Here's the drawing with two shaded views (mm, measured from the low corner). I have some questions. A direction names the side the tool comes from. Round coordinates to 2 decimals unless told otherwise and drop trailing zeros. Loops run counter-clockwise (first coordinate to the right, second up) from the corner with the lowest first, then second, coordinate; pieces in that order, holes last. Notation, with made-up numbers: (52.25, -38.5) - (109.25, -38.5) arc R11 cw to (109.25, -34.5) - close; hole circle Ø10 at (-25, 75). An arc over 180 degrees is marked (long way). Answer as CSV lines item,"result".
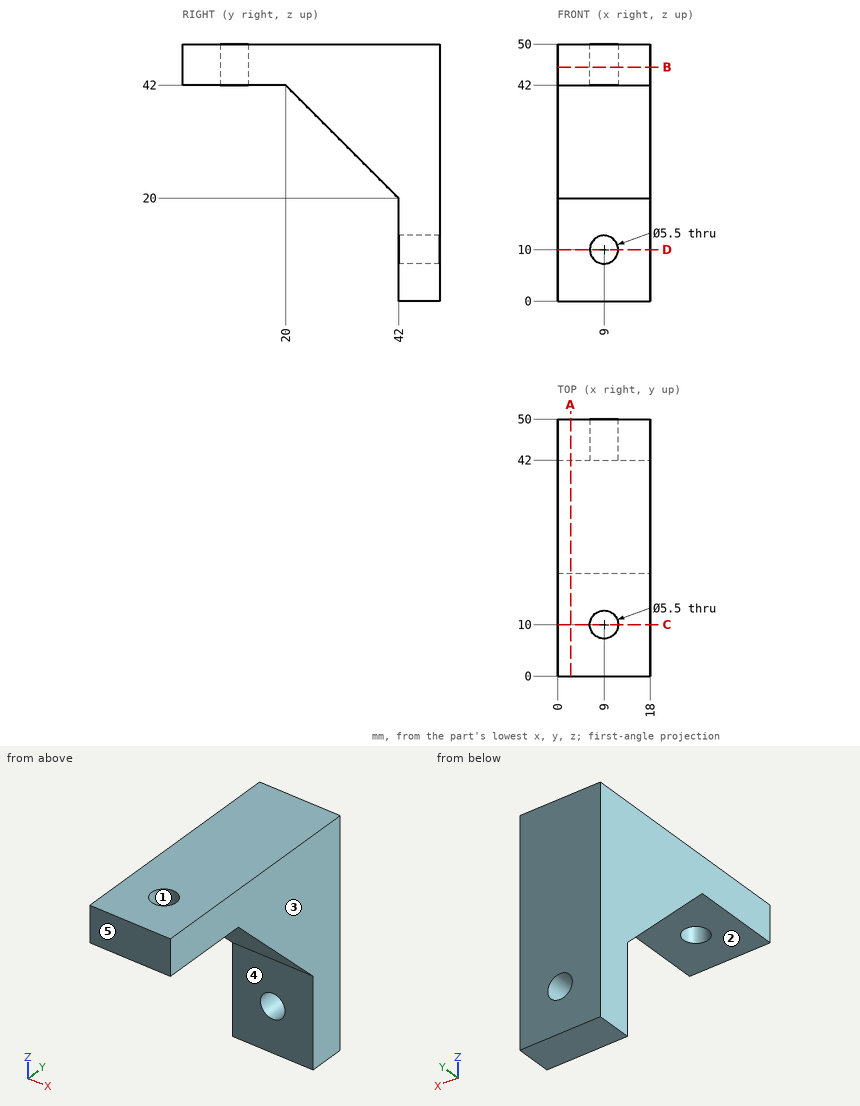
Q1. I'm going to push flat-ended pins straight in: pin 1 Ø1.5 at (x, y) = (12, 29.5) entering from -Z; pin 2 Ø9 at (x, y) = (9, 10) entering from -Z; pin 3 Ø6 at (x, z) = (9, 13.5) entering from -Y. Where does each tip first touch, or does it pass through?
Checks:
pin 1,"z = 31.75"
pin 2,"z = 42"
pin 3,"y = 42"
Q2. If I drill on line 1 along Y through (x, z) = (9, 46); line 2 along Y through (x, z) = (5, 11.5), over which ranges is the centre line in solid material (lowest first)? Write a range as [from, to].
Checks:
line 1,"[0, 7.25], [12.75, 50]"
line 2,"[42, 50]"
Q3. On a 3-axis mill with a long thin cutter (end or side, diameter ignored), from which of +Z, -Z, +X, -X, +Y, -Y can I reach the whole of each face in a straight line? I mean the marked faces 4 and 5. Say none if no direction works.
Checks:
face 4,"-Z, +X, -X, -Y"
face 5,"+Z, -Z, +X, -X, -Y"
Q4. Imagine slicing it at A-A (x = 2.5). Write out the boundary of the cut face in (y, z).
Checks:
outline,"(0, 42) - (20, 42) - (42, 20) - (42, 0) - (50, 0) - (50, 50) - (0, 50) - close"
Q5. Imagine slicing it at B-B (z = 45.5). Write out the boundary of the cut face in (x, y).
Checks:
outline,"(0, 0) - (18, 0) - (18, 50) - (0, 50) - close; hole circle Ø5.5 at (9, 10)"
Q6. Imagine slicing it at C-C (y = 10). Write out the boundary of the cut face in (x, z).
Checks:
outline,"(0, 42) - (6.25, 42) - (6.25, 50) - (0, 50) - close; (11.75, 42) - (18, 42) - (18, 50) - (11.75, 50) - close"
Q7. We'd pull the mould along X, two halves only. Please class the marked faces 1, 2 and 3: pulls with the +X half, pulls with the -X half, needs draft (parallel to the pull), parting line crosses it, or undercut.
Checks:
face 1,"undercut"
face 2,"needs draft"
face 3,"pulls with the +X half"
